Build history of the part. All positions in model axes, mm. Face numbers are marked on the shaded views. A direction names the side the tool comes from. Coordinates: 2 decimals unless noted, no trailing zeros. Loops run counter-clockwise (first coordinate to the right, second up) from the corner with the lowest first, then second, coordinate; pieces in that order, holes last.
Item 1: Drill centre lines: line 1 along Z through (x, y) = (0, 2.1); line 2 along Y through (x, z) = (4.5, 6.5); line 3 along Z through (x, y) = (-6, 26.4). Where is each one in solid material? Low to high.
Item 2: Mould opens along Z. For the marked faces 1, 2 and 3 say: released by +Z, released by -Z, zero draft, split by the parting line, or undercut.
Item 3: 3-axis set-ups, long thin cutter, end or side, ignore diameter. For the marked faces 4 and 5: which of +Z, -Z, +X, -X, +Y, -Y reach the whole face in a straight line?
Item 4: Flat gauge pins, fed straight in: pin 1 (4 mm diameter, centred on x = -9.5, z = -7, fed in from +Y); pin 2 (2.5 mm diameter, centred on x = 0, z = 6, fed in from +Y); pin 3 (6 mm diameter, centred on x = 2, z = -1, fed in from +Y); pin 4 (10 mm diameter, centred on y = 37.5, z = 1.5, fed in from -X). Where does each tip first touch, or does it go through?
Item 5: Cut at A-A (y = 14). List the corners of the cut face in (x, z).
Item 6: Cut at B-B (y = 23). List the corners of the cut face in (x, z), and give its area (3 significant figures).
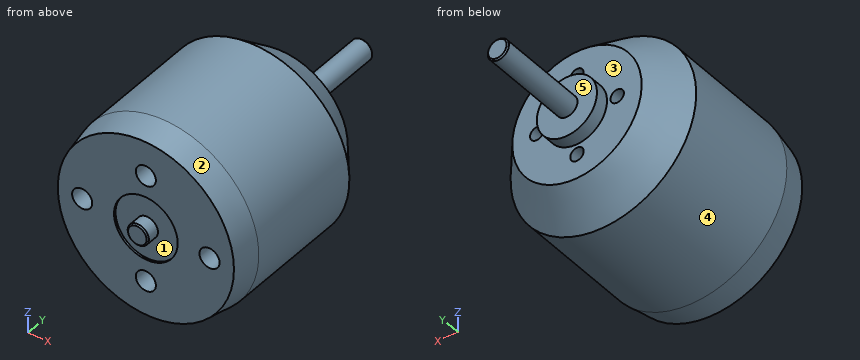
Autodesk Inventor part; units mm, degrees
ref_plane "YZ Plane" through (0, 0, 0) normal (1, 0, 0) x (0, 1, 0)
ref_plane "XZ Plane" through (0, 0, 0) normal (0, 1, 0) x (-1, 0, 0)
ref_plane "XY Plane" through (0, 0, 0) normal (0, 0, 1) x (1, 0, 0)
sketch "Sketch1" plane through (0, 0, 0) normal (0, 1, 0) x (-1, 0, 0)
  circle A0 centre (0, 0) radius 13.85
  dimension "d0" = 27.7
extrude "Extrusion1" add sketch "Sketch1" along normal blind 22
sketch "Sketch2" plane through (0, 0, 0) normal (1, 0, 0) x (0, 1, 0)
  line L0 (22, -13.85) -> (22, 13.85)
  line L1 (-4.4, 0) -> (26.4, 0)
  line L2 (22, -13.85) -> (27.25, -9.65)
  line L3 (27.25, -9.65) -> (27.25, 0)
  line L4 (22, 0) -> (22, -13.85)
  line L5 (27.25, 0) -> (22, 0)
  point P0 (0, 0)
  dimension "d3" = 5.25
  dimension "d6" = 9.65
revolve "Revolution1" add sketch "Sketch2" angle 360 about axis through (0, -10, 0) along (0, 1, 0)
chamfer "Chamfer1" distance 4 angle 10 1 edges at (13.85, 0, 0) measured on face at (1.6986, 14.6667, -13.7454)
sketch "Sketch3" plane through (0, 27.25, 0) normal (0, 1, 0) x (1, 0, 0)
  circle A0 centre (0, 0) radius 1.58
  dimension "d10" = 3.16
extrude "Extrusion2" add sketch "Sketch3" along normal blind 15.82
sketch "Sketch4" plane through (0, 27.25, 0) normal (0, 1, 0) x (1, 0, 0)
  circle A0 centre (0, 0) radius 4.485
  dimension "d13" = 8.97
extrude "Extrusion3" add sketch "Sketch4" along normal blind 2
sketch "Sketch5" plane through (0, 27.25, 0) normal (0, 1, 0) x (1, 0, 0)
  line L0 (0, 19.39) -> (0, -19.39)
  circle A0 centre (0, 6) radius 1
  point P0 (0, 0)
  dimension "d16" = 6
  dimension "d17" = 2
extrude "Extrusion4" cut sketch "Sketch5" against normal blind 3
thread "Thread1"
pattern_circular "Circular Pattern1" count 4 over 360 about axis through (0, -10, 0) along (0, 1, 0) of "Extrusion4"
sketch "Sketch6" plane through (0, 0, 0) normal (0, -1, 0) x (1, 0, 0)
  line L0 (-19.39, 0) -> (19.39, 0)
  line L1 (0, -19.39) -> (0, 19.39)
  circle A0 centre (9.5, 0) radius 1.5
  circle A1 centre (0, 8) radius 1.5
  circle A2 centre (-9.5, 0) radius 1.5
  circle A3 centre (0, -8) radius 1.5
  point P0 (0, 0)
  dimension "d25" = 9.5
  dimension "d26" = 8
  dimension "d27" = 3
extrude "Extrusion5" cut sketch "Sketch6" against normal blind 5
thread "Thread2"
thread "Thread3"
thread "Thread4"
thread "Thread5"
sketch "Sketch7" plane through (0, 0, 0) normal (0, -1, 0) x (1, 0, 0)
  circle A0 centre (0, 0) radius 4.75
  dimension "d38" = 9.5
extrude "Extrusion6" cut sketch "Sketch7" against normal blind 0.3
sketch "Sketch8" plane through (0, 0.3, 0) normal (0, -1, 0) x (1, 0, 0)
  circle A0 centre (0, 0) radius 1.58
extrude "Extrusion7" add sketch "Sketch8" along normal blind 2
chamfer "Chamfer2" distance 0.2 angle 45 2 edges at (-1.58, -1.7, 0) (-1.58, 43.07, 0)
properties part number "Brushless Motor"
Filled sheet:
1. line 1: z = -13.51 to -9.5, -6.5 to 6.5, 9.5 to 13.51
1. line 2: y = 0 to 27.25
1. line 3: z = -8.41 to -1, 1 to 8.41
2. face 1: undercut
2. face 2: split by the parting line
2. face 3: zero draft
3. face 4: +Y, -Y
3. face 5: +Y
4. pin 1: stops at y = 27.06
4. pin 2: stops at y = 27.25
4. pin 3: stops at y = 43.07
4. pin 4: stops at x = -1.58
5. outline: circle Ø27.7 at (0, 0)
6. outline: circle Ø26.1 at (0, 0)
6. area: 535 mm2
